Autodesk Inventor part; units mm, degrees
ref_plane "YZ Plane" through (0, 0, 0) normal (1, 0, 0) x (0, 1, 0)
ref_plane "XZ Plane" through (0, 0, 0) normal (0, 1, 0) x (-1, 0, 0)
ref_plane "XY Plane" through (0, 0, 0) normal (0, 0, 1) x (1, 0, 0)
sketch "Sketch1" plane through (0, 0, 0) normal (1, 0, 0) x (0, 1, 0)
  circle A0 centre (0, 0) radius 2.875
  arc A1 (0, 5) -> (0, -5) centre (0, 0) ccw
  line L0 (0, 5) -> (100, 5)
  line L1 (100, -5) -> (0, -5)
  arc A2 (100, -5) -> (100, 5) centre (100, 0) ccw
  circle A3 centre (100, 0) radius 3.1
  dimension "d0" = 5.75
  dimension "d1" = 10
  dimension "d3" = 100
  dimension "d5" = 6.2
  dimension "d27" = 5
extrude "Extrusion1" add sketch "Sketch1" along normal blind 3
ref_plane "Work Plane1" through (-2, 0, 0) normal (1, 0, 0) x (0, 0, -1)
equation "\"d27\" = 0.5 * d1"
properties part number "ServoLinkage_015"
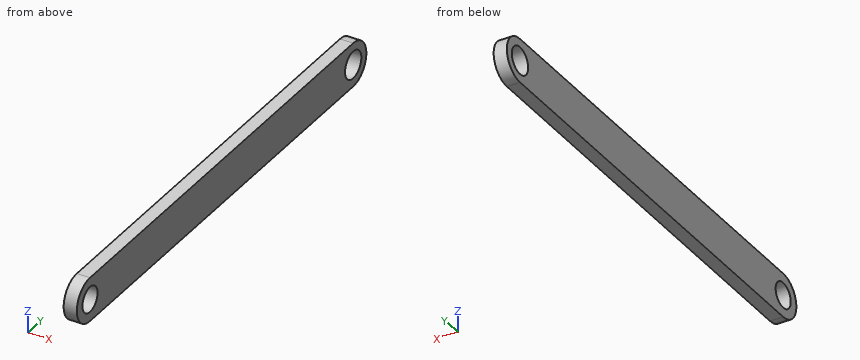
Here's how the part is built. I have some questions about the finished solid (model axes, mm). Coordinates: 2 decimals unless noted, no trailing zeros. Order: outer loops, then holes, each group sorted by start corner. A loop starts at its lowest first (then second) coordinate and runs counter-clockwise, first axis right, second up. Notation, with made-up numbers: (61.5, 14.25) - (101.5, 14.25) arc R18 cw to (101.5, 36.25) - close; hole circle Ø3 at (16, 29.25). An arc over 180 degrees is marked (long way). Use CSV: the item, a comma, the result in double quotes. Start each with the question number.
1. Suppose I cut it at A-A on z = 0. List the corners of the cut face in (x, y) for me (3 decimals), then the cut area to 3 significant figures.
2. Suppose I cut it at B-B on x = 1.7. List the corners of the cut face in (y, z) for me (3 decimals), then the cut area to 3 significant figures.
3. Please list where these lines run through material, in increasing order: line 1 (Y direction, x = 2.7, z = -0.25); line 2 (Z direction, x = 0.9, y = 100); line 3 (Z direction, x = 2.2, y = 0) (3 decimals). Write a range as from..to.
Output:
1,outline,"(0, -5) - (3, -5) - (3, -2.875) - (0, -2.875) - close; (0, 2.875) - (3, 2.875) - (3, 96.9) - (0, 96.9) - close; (0, 103.1) - (3, 103.1) - (3, 105) - (0, 105) - close"
1,area,"294 mm2"
2,outline,"(0, -5) - (100, -5) arc R5 ccw to (100, 5) - (0, 5) arc R5 ccw to start; hole circle Ø5.75 at (0, 0); hole circle Ø6.2 at (100, 0)"
2,area,"1,020 mm2"
3,line 1,"y = -4.99..-2.86, 2.86..96.91, 103.09..104.99"
3,line 2,"z = -5..-3.1, 3.1..5"
3,line 3,"z = -5..-2.875, 2.875..5"
